from build123d import *

# Parameters (mm, degrees)
SKETCH_1_W           = 300
SKETCH_1_H           = 300
EXTRUDE_1_DEPTH      = 5
CUT_EXTRUDE_3_DEPTH  = 10
CUT_EXTRUDE_5_DEPTH  = 10
SKETCH_7_OUTSIDE_W   = 373.028
SKETCH_7_OUTSIDE_H   = 263.028
SKETCH_7_OUTSIDE_W_2 = 283
SKETCH_7_OUTSIDE_H_2 = 188
CUT_EXTRUDE_6_DEPTH  = 10
FILLET_1_R           = 10
SKETCH_8_R           = 1.5
CUT_EXTRUDE_7_DEPTH  = 200
SKETCH_9_R           = 1.5
CUT_EXTRUDE_8_DEPTH  = 200
SKETCH_10_W          = 140
SKETCH_10_H          = 50
EXTRUDE_2_DEPTH      = 5
FILLET_2_R           = 10


with BuildPart() as part:
    # 草图1 → 凸台-拉伸1 (new body)
    with BuildSketch(Plane(origin=(0, 0, 0), x_dir=(1, 0, 0), z_dir=(0, 1, 0))):
        Rectangle(SKETCH_1_W, SKETCH_1_H)
    extrude(amount=EXTRUDE_1_DEPTH)

    # 草图4 → 切除-拉伸3 (cut)
    with BuildSketch(Plane(origin=(0, 5, 0), x_dir=(1, 0, 0), z_dir=(0, 1, 0))):
        Polygon((-88.251311829, 95), (84.324863402, 95), (73.252498177, 170.696662895), (-48.543519298, 170.696662895), align=None)
        Polygon((-81.835862219, -95), (-68.397415564, -170.764406983), (34.942066678, -175.273207327), (78.78868079, -129.283443823), (78.78868079, -95), align=None)
    extrude(amount=-CUT_EXTRUDE_3_DEPTH, mode=Mode.SUBTRACT)

    # 草图6 → 切除-拉伸5 (cut)
    with BuildSketch(Plane(origin=(0, 5, 0), x_dir=(1, 0, 0), z_dir=(0, 1, 0))):
        Polygon((-88.251311829, 95), (233.509150227, 95), (223.865704495, 204.923221807), (-177.714928491, 215.944302643), (-226.620974704, 137.419101682), (-226.620974704, 114.688122456), (-226.620974704, 95), align=None)
        Polygon((-81.835862219, -95), (223.865704495, -95), (223.865704495, -205.612039359), (-238.330873093, -205.612039359), (-238.330873093, -95), align=None)
    extrude(amount=-CUT_EXTRUDE_5_DEPTH, mode=Mode.SUBTRACT)

    # 草图7 outside → 切除-拉伸6 (cut)
    with BuildSketch(Plane(origin=(0, 5, 0), x_dir=(1, 0, 0), z_dir=(0, 1, 0))):
        Rectangle(SKETCH_7_OUTSIDE_W, SKETCH_7_OUTSIDE_H)
        Rectangle(SKETCH_7_OUTSIDE_W_2, SKETCH_7_OUTSIDE_H_2, mode=Mode.SUBTRACT)
    extrude(amount=-CUT_EXTRUDE_6_DEPTH, mode=Mode.SUBTRACT)

    # 圆角1
    fillet_1_edges = [part.edges().sort_by_distance(p)[0] for p in [
        (-141.5, 2.5, -94),
        (141.5, 2.5, -94),
        (141.5, 2.5, 94),
        (-141.5, 2.5, 94),
    ]]
    fillet(fillet_1_edges, radius=FILLET_1_R)

    # 草图8 → 切除-拉伸7 (cut)
    with BuildSketch(Plane(origin=(0, 5, 0), x_dir=(1, 0, 0), z_dir=(0, 1, 0))):
        with Locations(Location((-132.5, 0, 0), (0, 0, 270))):
            Circle(SKETCH_8_R)
        with Locations(Location((132.5, 0, 0), (0, 0, 270))):
            Circle(SKETCH_8_R)
    extrude(amount=-CUT_EXTRUDE_7_DEPTH, mode=Mode.SUBTRACT)

    # 草图9 → 切除-拉伸8 (cut)
    with BuildSketch(Plane(origin=(0, 5, 0), x_dir=(1, 0, 0), z_dir=(0, 1, 0))):
        with Locations(Location((-50, 90, 0), (0, 0, 270))):
            Circle(SKETCH_9_R)
        with Locations(Location((50, 90, 0), (0, 0, 270))):
            Circle(SKETCH_9_R)
    cut_extrude_8 = extrude(amount=-CUT_EXTRUDE_8_DEPTH, mode=Mode.SUBTRACT)

    # 镜向1: 切除-拉伸8 across plane
    add(cut_extrude_8.mirror(Plane.XY), mode=Mode.SUBTRACT)

    # 草图10 → 凸台-拉伸2 (add)
    with BuildSketch(Plane(origin=(0, 5, 0), x_dir=(1, 0, 0), z_dir=(0, 1, 0))):
        with Locations((0, -119)):
            Rectangle(SKETCH_10_W, SKETCH_10_H)
        with Locations((0, 119)):
            Rectangle(SKETCH_10_W, SKETCH_10_H)
    extrude(amount=-EXTRUDE_2_DEPTH)

    # 圆角2
    fillet_2_edges = [part.edges().sort_by_distance(p)[0] for p in [
        (-70, 2.5, 144),
        (-70, 2.5, 94),
        (70, 2.5, 94),
        (70, 2.5, 144),
        (70, 2.5, -94),
        (-70, 2.5, -94),
        (-70, 2.5, -144),
        (70, 2.5, -144),
    ]]
    fillet(fillet_2_edges, radius=FILLET_2_R)


solid = part.part
Geometry check sheet. Reference: the model listing, model coordinates, mm. Give positions to 0.01 mm unless a question says otherwise; leave off trailing zeros.
1) Go/stop test with flat-tipped pins: pin 1 Ø2.5 at (y, z) = (3.5, -123) entering from +X; pin 2 Ø1.5 at (x, y) = (116.5, 3.5) entering from -Z; pin 3 Ø1.5 at (y, z) = (3, 120.5) entering from -X. Record where each tip stops, or that it passes through.
Values follow:
pin 1: stops at x = 70
pin 2: stops at z = -94
pin 3: stops at x = -70
2) Cross-section at A-A (y = 2.05). Count the separate pieces of the cut face and the enclosed holes in it, plus the area to 3 significant figures.
Values follow:
separate pieces: 1
enclosed holes: 6
area: 67,100 mm2
3) Thickness scan on line 1 (X direction, y = 2.65, z = 0); line 2 (Z direction, x = -132.5, y = 1.9); line 3 (X direction, y = 1.8, z = 90). Record the ranges inside material, lowest first.
Values follow:
line 1: x = -141.5 to -134, -131 to 131, 134 to 141.5
line 2: z = -93.95 to -1.5, 1.5 to 93.95
line 3: x = -139.5 to -51.5, -48.5 to 48.5, 51.5 to 139.5
4) Release check for a two-part mould opening along Z. For faces 1 (the face through (-2, 5, -2)), 2 (the face through (-67.15, 2.46, 140.99)), 3 (the face through (67.15, 2.46, -140.99)) record: released by +Z, released by -Z, zero draft, split by the parting line, or undercut.
Values follow:
face 1: zero draft
face 2: released by +Z
face 3: released by -Z
